from build123d import *

# Parameters (mm, degrees)
BOSS_EXTRUDE1_DEPTH = 15.3
SKETCH2_R           = 9.3
CUT_EXTRUDE1_DEPTH  = 3.1
BOSS_EXTRUDE2_START = 8
BOSS_EXTRUDE2_DEPTH = 8
BOSS_EXTRUDE3_START = 3
SKETCH4_R           = 2
BOSS_EXTRUDE3_DEPTH = 3
BOSS_EXTRUDE4_START = 1.8
SKETCH5_R           = 4
SKETCH5_R_2         = 2
BOSS_EXTRUDE4_DEPTH = 1.8
FILLET1_R           = 4
FILLET2_R           = 1
CUT_EXTRUDE2_START  = -2.2
SKETCH7_R           = 2
CUT_EXTRUDE2_DEPTH  = 2.2
SKETCH9_R           = 21.205552102
CUT_EXTRUDE4_DEPTH  = 23.3
SKETCH8_W           = 42.45562683
SKETCH8_H           = 26.950518874
CUT_EXTRUDE5_DEPTH  = 21.71696165
CUT_EXTRUDE6_DEPTH  = 10


with BuildPart() as part:
    # Sketch1 → Boss-Extrude1 (new body)
    with BuildSketch(Plane.XY):
        with BuildLine():
            Line((-8.55, 0), (-16.55, 0))
            Line((-16.55, 0), (-16.55, 3.5))
            Line((-16.55, 3.5), (-10.95445115, 3.5))
            ThreePointArc((-10.95445115, 3.5), (0, 11.5), (10.95445115, 3.5))
            Line((10.95445115, 3.5), (16.55, 3.5))
            Line((16.55, 3.5), (16.55, 0))
            Line((16.55, 0), (8.55, 0))
            ThreePointArc((8.55, 0), (0, 8.55), (-8.55, 0))
        make_face()
    extrude(amount=-BOSS_EXTRUDE1_DEPTH)

    # Sketch2 → Cut-Extrude1 (cut)
    with BuildSketch(Plane.XY.offset(-6.3)):
        Circle(SKETCH2_R)
    extrude(amount=-CUT_EXTRUDE1_DEPTH, mode=Mode.SUBTRACT)

    # Sketch3 → Boss-Extrude2 (add)
    with BuildSketch(Plane.XY.offset(BOSS_EXTRUDE2_START)):
        with BuildLine():
            Line((-10.25, 0), (-16.55, 0))
            Line((-16.55, 0), (-16.55, 3.5))
            Line((-16.55, 3.5), (-10.95445115, 3.5))
            ThreePointArc((-10.95445115, 3.5), (0, 11.5), (10.95445115, 3.5))
            Line((10.95445115, 3.5), (16.55, 3.5))
            Line((16.55, 3.5), (16.55, 0))
            Line((16.55, 0), (10.25, 0))
            ThreePointArc((10.25, 0), (0, 10.25), (-10.25, 0))
        make_face()
    extrude(amount=-BOSS_EXTRUDE2_DEPTH)

    # Sketch4 → Boss-Extrude3 (add)
    with BuildSketch(Plane.XY.offset(8).offset(BOSS_EXTRUDE3_START)):
        with BuildLine():
            Line((-11.5, 0), (-16.55, 0))
            Line((-16.55, 0), (-16.55, 3.5))
            Line((-16.55, 3.5), (-10.95445115, 3.5))
            ThreePointArc((-10.95445115, 3.5), (0, 11.5), (10.95445115, 3.5))
            Line((10.95445115, 3.5), (16.55, 3.5))
            Line((16.55, 3.5), (16.55, 0))
            Line((16.55, 0), (11.5, 0))
            ThreePointArc((11.5, 0), (0, -11.5), (-11.5, 0))
        make_face()
        Circle(SKETCH4_R, mode=Mode.SUBTRACT)
    extrude(amount=-BOSS_EXTRUDE3_DEPTH)

    # Sketch5 → Boss-Extrude4 (add)
    with BuildSketch(Plane.XY.offset(11).offset(BOSS_EXTRUDE4_START)):
        Circle(SKETCH5_R)
        Circle(SKETCH5_R_2, mode=Mode.SUBTRACT)
    extrude(amount=-BOSS_EXTRUDE4_DEPTH)

    # Fillet1
    # the kernel refuses this fillet: 4 mm, written as the material it adds along each edge
    with BuildSketch(Plane(origin=(0, 0, 11), x_dir=(1, 0, 0), z_dir=(0, -1, 0))) as fillet1_piece_1:
        with BuildLine():
            CenterArc((7.340658618, 4), FILLET1_R, 213.367012969, 56.632987031)
            Line((7.340658618, 0), (7.340658618, -0.08))
            Line((7.340658618, -0.08), (4, -0.08))
            Line((4, -0.08), (3.92, 0))
            ThreePointArc((3.92, 0), (3.92, 0.9), (3.933186828, 1.756))
            Line((3.933186828, 1.756), (4, 1.8))
        make_face()
    revolve(axis=Axis((0, 0, 11), (0, 0, 1)))

    # Fillet2
    fillet2_edges = [part.edges().sort_by_distance(p)[0] for p in [
        (0, 10.25, 8),
    ]]
    fillet(fillet2_edges, radius=FILLET2_R)

    # Sketch7 → Cut-Extrude2 (cut)
    with BuildSketch(Plane(origin=(0, 0, 8), x_dir=(-1, 0, 0), z_dir=(0, 0, -1)).offset(CUT_EXTRUDE2_START)):
        Polygon((5.55, 2.65), (5.55, -6.55), (3.15, -6.55), (3.15, -10.55), (-3.15, -10.55), (-6.775322586, -10.55), (-8.767406073, -8.55), (-3.15, -8.55), (-3.15, -6.55), (-5.55, -6.55), (-5.55, 2.65), (-2.65, 5.55), (2.65, 5.55), align=None)
        Circle(SKETCH7_R, mode=Mode.SUBTRACT)
    extrude(amount=CUT_EXTRUDE2_DEPTH, mode=Mode.SUBTRACT)

    # Sketch9 → Cut-Extrude4 (cut)
    with BuildSketch(Plane(origin=(0, 0, 8), x_dir=(-1, 0, 0), z_dir=(0, 0, -1))):
        Circle(SKETCH9_R)
    extrude(amount=CUT_EXTRUDE4_DEPTH, mode=Mode.SUBTRACT)

    # Sketch8 → Cut-Extrude5 (cut, through all)
    with BuildSketch(Plane(origin=(0, 0, 8), x_dir=(-1, 0, 0), z_dir=(0, 0, -1))):
        Rectangle(SKETCH8_W, SKETCH8_H)
        with BuildLine():
            Line((11.5, 0), (9.45, 0))
            ThreePointArc((9.45, 0), (0, 9.45), (-9.45, 0))
            Line((-9.45, 0), (-11.5, 0))
            ThreePointArc((-11.5, 0), (0, -11.5), (11.5, 0))
        make_face(mode=Mode.SUBTRACT)
    extrude(amount=-CUT_EXTRUDE5_DEPTH, mode=Mode.SUBTRACT)

    # Sketch10 → Cut-Extrude6 (cut)
    with BuildSketch(Plane.XY.offset(11)):
        with BuildLine():
            Line((-10.789833042, 0), (-10.789833042, -3.978630786))
            ThreePointArc((-10.789833042, -3.978630786), (-11.321066204, -2.020757286), (-11.5, 0))
            Line((-11.5, 0), (-10.789833042, 0))
        make_face()
        with BuildLine():
            Line((10.95445115, 0), (10.95445115, -3.5))
            ThreePointArc((10.95445115, -3.5), (11.362794292, -1.771131245), (11.5, 0))
            Line((11.5, 0), (10.95445115, 0))
        make_face()
    extrude(amount=-CUT_EXTRUDE6_DEPTH, mode=Mode.SUBTRACT)


solid = part.part
For this review, take the finished solid that the model builds, in its own axes (mm). A direction names the side the tool comes from. Give positions to 0.01 mm unless a question says otherwise; leave off trailing zeros. Loops run counter-clockwise (first coordinate to the right, second up) from the corner with the lowest first, then second, coordinate; pieces in that order, holes last. Notation, with made-up numbers: (-1, -37) - (54, -37) arc R12 ccw to (54, -21) - close; hole circle Ø6 at (-29.5, 67). An arc over 180 degrees is marked (long way). Write each question's results on one line, items separated by ' | '.
(1) Draft analysis for pull direction X (two halves, no side actions). For faces 1 (the flat face through (10.954, -2, 10)), 2 (the flat face through (-10, 0, 9)), 3 (the flat face through (-4, -6.55, 9)), 4 (the flat face through (-10.79, -2, 10)), state which applies: +X half, -X half, draft (parallel to the pull), parting line (faces both ways), or undercut.
Conclusion:
face 1: +X half | face 2: draft | face 3: undercut | face 4: -X half
(2) Take a section at A-A (x = 0). Give the boundary of the cut face in (y, z), then the cut area to 3 significant figures.
Conclusion:
outline: (-11.5, 8) - (-10.55, 8) - (-10.55, 10.2) - (-2, 10.2) - (-2, 12.8) - (-4, 12.8) arc R4 cw to (-7.34, 11) - (-11.5, 11) - close; (2, 10.2) - (5.55, 10.2) - (5.55, 8) - (9.45, 8) - (9.45, 11) - (7.34, 11) arc R4 cw to (4, 12.8) - (2, 12.8) - close | area: 35.0 mm^2
(3) Take a section at D-D (x = 8.25). Give the boundary of the cut face in (y, z), then the cut area to 3 significant figures.
Conclusion:
outline: (-8.01, 8) - (4.61, 8) - (4.61, 11) - (-8.01, 11) - close | area: 37.9 mm^2
(4) Take a section at B-B (z = 8.95). Give the boundary of the cut face in (x, y).
Conclusion:
outline: (-10.79, -3.98) arc R11.5 ccw to (4.58, -10.55) - (-3.15, -10.55) - (-3.15, -6.55) - (-5.55, -6.55) - (-5.55, 2.65) - (-2.65, 5.55) - (2.65, 5.55) - (5.55, 2.65) - (5.55, -6.55) - (3.15, -6.55) - (3.15, -8.55) - (7.69, -8.55) arc R11.5 ccw to (10.95, -3.5) - (10.95, 0) - (9.45, 0) arc R9.45 ccw to (-9.45, 0) - (-10.79, 0) - close
(5) For line 1 along Z through (x, y) = (2, 7.25); line 2 along X through (y, z) = (-3.5, 8.3); line 3 along Y through (x, z) = (0, 11.4), list the stretches that pass through material, from the lowest coordinate up.
Conclusion:
line 1: 8 to 11 | line 2: -10.79 to -5.55, 5.55 to 10.95 | line 3: -5.6 to -2, 2 to 5.6
(6) For faces 5 (the flat face through (-5, 4, 8)), 6 (the flat face through (5, -8.55, 9)), 7 (the flat face through (0, -8, 11)), 8 (the flat face through (-4.1, 4.1, 9.1)), 9 (the flat face through (10, 0, 9)), list the 3-axis set-ups (+Z, -Z, +X, -X, +Y, -Y) from which the entire face can be reached by the end or side of a thin tool; tool diameter is ignored.
Conclusion:
face 5: -Z, +X, -X, +Y, -Y | face 6: -Z, +X | face 7: +Z | face 8: -Z | face 9: +Z, -Z, +X, +Y
(7) For pin 1 Ø2.5 at (x, z) = (5, 9) entering from -Y; pin 2 Ø0.7 at (x, z) = (2.5, 9) entering from +Y; pin 3 Ø1.7 at (x, z) = (10.5, 9.5) entering from +Y; pin 4 Ø1.8 at (x, z) = (-1, 9) entering from -Y, all flat-tipped, find the tip position at first contact; note any pin that passes through.
Conclusion:
pin 1: y = -10.87 | pin 2: y = 9.2 | pin 3: y = 0 | pin 4: y = -11.5
(8) Take a section at C-C (y = -9.5). Give the boundary of the cut face in (x, z), then the cut area to 3 significant figures.
Conclusion:
outline: (-6.48, 8) - (-3.15, 8) - (-3.15, 10.2) - (6.48, 10.2) - (6.48, 11) - (-6.48, 11) - close | area: 17.7 mm^2
